The listing builds one solid part. Answer for the finished solid, in the listing's coordinates (mm). A direction names the side the tool comes from. Coordinates: 2 decimals unless noted, no trailing zeros. Order: outer loops, then holes, each group sorted by start corner. A loop starts at its lowest first (then second) coordinate and runs counter-clockwise, first axis right, second up. Notation, with made-up numbers: (59.5, -31.75) -> (92.5, -31.75) arc R25 cw to (92.5, 1.25) -> close; hole circle Ø4 at (61, 37.25). An arc over 180 degrees is marked (long way). Answer in a Markdown table with one row per item.
```python
from build123d import *

# Parameters (mm, degrees)
RESSALTO_EXTRUS_O1_DEPTH = 5


with BuildPart() as part:
    # Model → Ressalto-extrusão1 (new body)
    with BuildSketch(Plane.XY):
        with BuildLine():
            Line((-182.000002727, 45.000001207), (-182.000002727, 54.000000805))
            Line((-182.000002727, 54.000000805), (-187.000002816, 54.000000805))
            Line((-187.000002816, 54.000000805), (-187.000002816, 64.000000954))
            Line((-187.000002816, 64.000000954), (-182.000002727, 64.000000954))
            Line((-182.000002727, 64.000000954), (-182.000002727, 68.000001045))
            Line((-182.000002727, 68.000001045), (-175.200002727, 68.000001045))
            Line((-175.200002727, 68.000001045), (-175.200002727, 66.800001045))
            Line((-175.200002727, 66.800001045), (-172.800002727, 66.800001045))
            Line((-172.800002727, 66.800001045), (-172.800002727, 68.000001045))
            Line((-172.800002727, 68.000001045), (-171.000002727, 68.000001045))
            Line((-171.000002727, 68.000001045), (-171.000002727, 71.000001026))
            Line((-171.000002727, 71.000001026), (-172.800002727, 71.000001026))
            Line((-172.800002727, 71.000001026), (-172.800002727, 72.200001026))
            Line((-172.800002727, 72.200001026), (-175.200002727, 72.200001026))
            Line((-175.200002727, 72.200001026), (-175.200002727, 71.000001026))
            Line((-175.200002727, 71.000001026), (-182.000002727, 71.000001026))
            Line((-182.000002727, 71.000001026), (-182.000002727, 75.000001118))
            Line((-182.000002727, 75.000001118), (-187.000002816, 75.000001118))
            Line((-187.000002816, 75.000001118), (-187.000002816, 85.000001267))
            Line((-187.000002816, 85.000001267), (-182.000002727, 85.000001267))
            Line((-182.000002727, 85.000001267), (-182.000002727, 112.000001058))
            Line((-182.000002727, 112.000001058), (-175.200002727, 112.000001058))
            Line((-175.200002727, 112.000001058), (-175.200002727, 110.800001058))
            Line((-175.200002727, 110.800001058), (-172.800002727, 110.800001058))
            Line((-172.800002727, 110.800001058), (-172.800002727, 112.000001058))
            Line((-172.800002727, 112.000001058), (-171.000002727, 112.000001058))
            Line((-171.000002727, 112.000001058), (-171.000002727, 115.00000104))
            Line((-171.000002727, 115.00000104), (-172.800002727, 115.00000104))
            Line((-172.800002727, 115.00000104), (-172.800002727, 116.20000104))
            Line((-172.800002727, 116.20000104), (-175.200002727, 116.20000104))
            Line((-175.200002727, 116.20000104), (-175.200002727, 115.00000104))
            Line((-175.200002727, 115.00000104), (-182.000002727, 115.00000104))
            Line((-182.000002727, 115.00000104), (-182.000002727, 131.000001952))
            Line((-182.000002727, 131.000001952), (-187.000002816, 131.000001952))
            Line((-187.000002816, 131.000001952), (-187.000002816, 139.000002071))
            Line((-187.000002816, 139.000002071), (-182.000002727, 139.000002071))
            Line((-182.000002727, 139.000002071), (-182.000002727, 143.000002162))
            ThreePointArc((-182.000002727, 143.000002162), (-181.707109508, 143.707108943), (-181.000002727, 144.000002162))
            Line((-181.000002727, 144.000002162), (-180.698724383, 144.000002162))
            ThreePointArc((-180.698724383, 144.000002162), (-177.250425834, 143.20301546), (-174.467200153, 141.016784571))
            ThreePointArc((-174.467200153, 141.016784571), (-157.893266413, 94.000001418), (-174.467200151, 46.983218264))
            ThreePointArc((-174.467200151, 46.983218264), (-177.245806987, 44.787339393), (-180.698724383, 44.000001207))
            Line((-180.698724383, 44.000001207), (-181.000002727, 44.000001207))
            ThreePointArc((-181.000002727, 44.000001207), (-181.707109508, 44.292894425), (-182.000002727, 45.000001207))
        make_face()
    extrude(amount=RESSALTO_EXTRUS_O1_DEPTH)


solid = part.part
```
(1) A cutting plane is placed at A-A, the plane x = -166.75. Determine the outline of the cut face in (y, z), then the cut area to 3 significant figures.
Check values:
| item | result |
|---|---|
| outline | (58.65, 0) -> (129.35, 0) -> (129.35, 5) -> (58.65, 5) -> close |
| area | 354 mm² |
(2) Which of the six approach directions +Z, -Z, +X, -X, +Y, -Y give full straight-line access (tool end or side, diameter ignored) to faces 5 (the flat face through (-185, 139, 2)), 6 (the cylindrical face through (-177.296, 143.224, 2.465)), 7 (the flat face through (-174, 116.2, 2)), 8 (the flat face through (-171, 69, 2))?
Check values:
| item | result |
|---|---|
| face 5 | +Z, -Z, -X, +Y |
| face 6 | +Z, -Z, +X, +Y |
| face 7 | +Z, -Z |
| face 8 | +Z, -Z, -X |
(3) Find the intervals of material crossed by line 1 along Y through (x, z) = (-185, 0.9); line 2 along Y through (x, z) = (-179, 2.9); line 3 along X through (y, z) = (56.5, 4.65), in increasing order. Write a range as from..to.
Check values:
| item | result |
|---|---|
| line 1 | 54..64, 75..85, 131..139 |
| line 2 | 44.18..68, 71..112, 115..143.81 |
| line 3 | -187..-167.95 |
(4) A cutting plane is placed at B-B, the plane y = 89. Determine the outline of the cut face in (x, z).
Check values:
| item | result |
|---|---|
| outline | (-182, 0) -> (-158.06, 0) -> (-158.06, 5) -> (-182, 5) -> close |
(5) Flat-ended cylindrical pins translate along their axes: pin 1 (2 mm diameter, centred on x = -172.5, z = 1.5, fed in from +Y); pin 2 (1.5 mm diameter, centred on x = -183.5, z = 3.5, fed in from +Y); pin 3 (1 mm diameter, centred on y = 116, z = 2.5, fed in from +X). Find the tip coordinate at first contact, or state that the pin passes through.
Check values:
| item | result |
|---|---|
| pin 1 | y = 139.79 |
| pin 2 | y = 139 |
| pin 3 | x = -161.04 |
(6) For a pull along X with two mould halves and no side action, classify faces 1 (the flat face through (-174, 110.8, 2)), 2 (the flat face through (-172, 115, 2)), 3 (the flat face through (-187, 135, 2)), 4 (the flat face through (-174, 72.2, 2)) as released by +X, released by -X, zero draft, split by the parting line, or undercut.
Check values:
| item | result |
|---|---|
| face 1 | undercut |
| face 2 | zero draft |
| face 3 | released by -X |
| face 4 | undercut |
